Could you check a few things on this drawing? It's one solid part, dimensions in mm from its lowest x, y, z. A direction names the side the tool comes from. Give positions to 0.01 mm unless a question says otherwise; leave off trailing zeros. Loops run counter-clockwise (first coordinate to the right, second up) from the corner with the lowest first, then second, coordinate; pieces in that order, holes last. Notation, with made-up numbers: (23, 84.5) - (50, 84.5) arc R29 cw to (50, 107.5) - close; hole circle Ø2 at (47, -40). An arc over 180 degrees is marked (long way). Use CSV: the item, a comma, the result in double quotes.
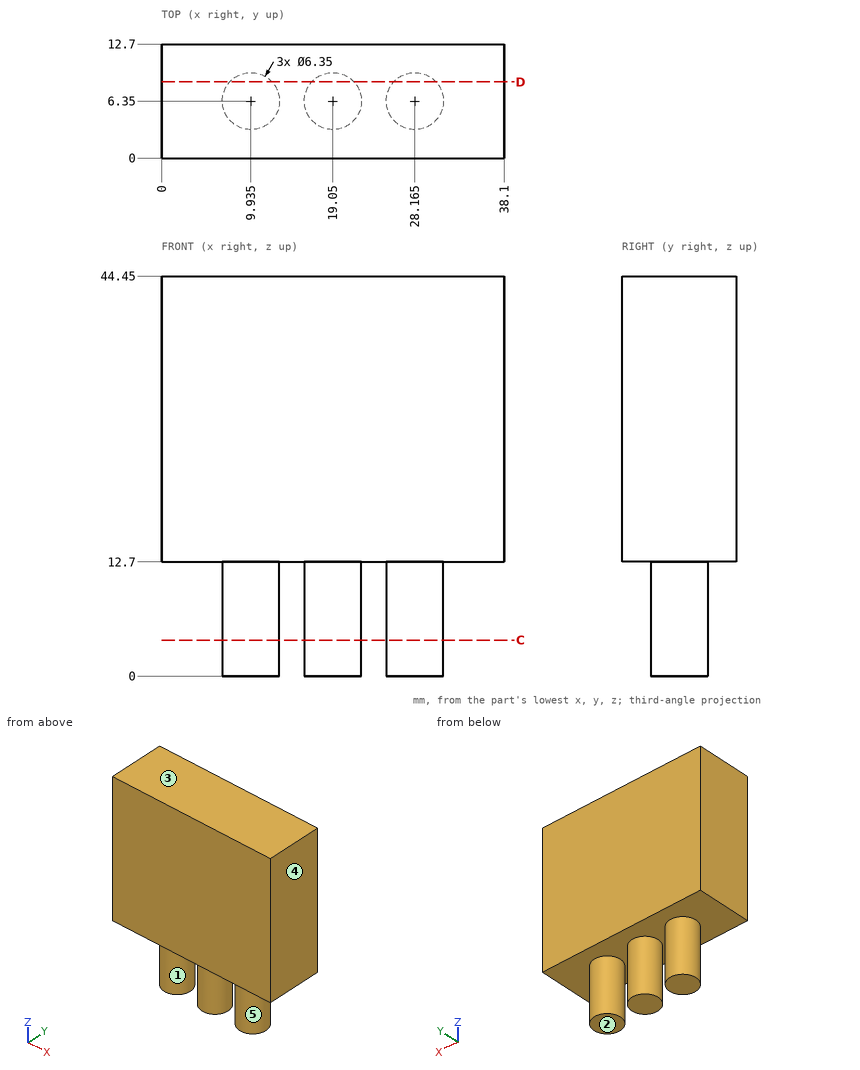
1) We'd pull the mould along X, two halves only. Please class the marked faces 3, 4 and 5: +X half, -X half, draft (parallel to the pull), parting line (faces both ways), or undercut.
Answer below:
face 3,"draft"
face 4,"+X half"
face 5,"undercut"
2) I'm going to push flat-ended pins straight in: P1, Ø6, axis at x = 23.5, y = 1.5, coming from the -Z side; P2, Ø4, axis at y = 5, z = 9.5, coming from the +X side; P3, Ø2, axis at x = 19, z = 10, coming from the +Y side (3 decimals). Where does each tip first touch, or does it pass through?
Answer below:
P1,"stops at z = 12.7"
P2,"stops at x = 31.34"
P3,"stops at y = 9.525"
3) Which directions (+Z, -Z, +X, -X, +Y, -Y) give clear straight access to the entire face, cutting with the end or side of a thin tool? Please do the marked faces 1 and 2.
Answer below:
face 1,"-Z"
face 2,"-Z, +X, -X, +Y, -Y"
4) Suppose I cut it at C-C (z = 4). State how many separate pieces and enclosed holes the cut face has.
Answer below:
separate pieces,"3"
enclosed holes,"0"
5) Suppose I cut it at D-D (y = 8.5). Please give me the cut outline in (x, z).
Answer below:
outline,"(0, 12.7) - (7.6, 12.7) - (7.6, 0) - (12.27, 0) - (12.27, 12.7) - (16.71, 12.7) - (16.71, 0) - (21.39, 0) - (21.39, 12.7) - (25.83, 12.7) - (25.83, 0) - (30.5, 0) - (30.5, 12.7) - (38.1, 12.7) - (38.1, 44.45) - (0, 44.45) - close"
6) I need wall thicknesses on line 1 along X through (y, z) = (8.5, 8.5) (1 decimal); line 2 along Z through (x, y) = (23.5, 6.75); line 3 along Y through (x, z) = (28, 7). Which ranges of each line are inside material? Lowest first, please.
Answer below:
line 1,"x = 7.6 to 12.3, 16.7 to 21.4, 25.8 to 30.5"
line 2,"z = 12.7 to 44.45"
line 3,"y = 3.18 to 9.52"
